Can you work these out from the drawing? Everything is in mm from the part's minimum corner. A direction names the side the tool comes from. Round coordinates to 2 decimals unless told otherwise and drop trailing zeros. Loops run counter-clockwise (first coordinate to the right, second up) from the corner with the lowest first, then second, coordinate; pieces in that order, holes last. Notation, with made-up numbers: M -30,20.5 L -8,20.5 A28 ccw -8,56.5 Z; hole C 66.25,68 d10. An arc over 180 degrees is marked long. Use a Markdown table: item, result.
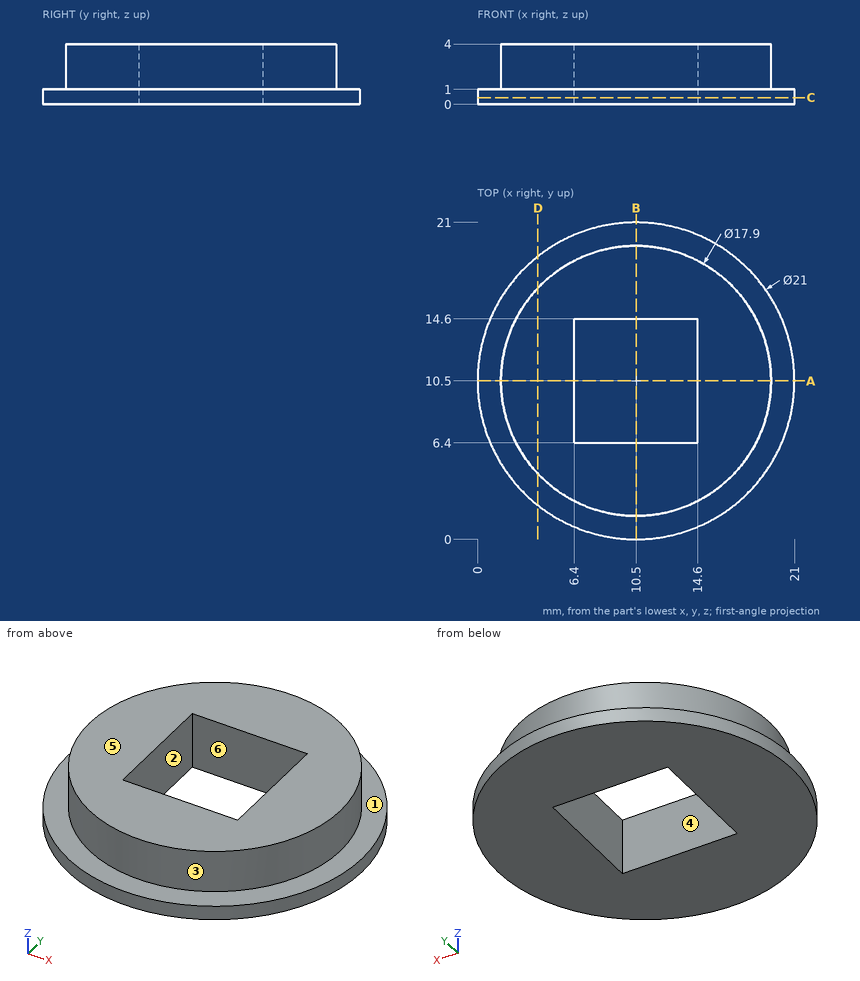
1. We'd pull the mould along X, two halves only. Please class the marked faces 1, 2, 3 and 4: +X half, -X half, draft (parallel to the pull), parting line (faces both ways), or undercut.
Answer sheet:
| item | result |
|---|---|
| face 1 | draft |
| face 2 | undercut |
| face 3 | parting line |
| face 4 | undercut |
2. For pin 1 Ø1.5 at (x, z) = (13, 1) entering from -Y; pin 2 Ø2 at (y, z) = (8.5, 1) entering from -X; pin 3 Ø2 at (x, z) = (18.5, 1.5) entering from +Y, each with a flat end and sliding along its axis, tell me the tip position at first contact or that it passes through.
Answer sheet:
| item | result |
|---|---|
| pin 1 | y = 0.15 |
| pin 2 | x = 0.05 |
| pin 3 | y = 18.2 |
3. Imagine slicing it at C-C, the plane z = 0.45. Write out the boundary of the cut face in (x, y).
Answer sheet:
| item | result |
|---|---|
| outline | C 10.5,10.5 d21; hole M 6.4,6.4 L 14.6,6.4 L 14.6,14.6 L 6.4,14.6 Z |
4. Imagine slicing it at D-D, the plane x = 4. Write out the boundary of the cut face in (y, z), then the cut area to 3 significant figures.
Answer sheet:
| item | result |
|---|---|
| outline | M 2.25,0 L 18.75,0 L 18.75,1 L 16.65,1 L 16.65,4 L 4.35,4 L 4.35,1 L 2.25,1 Z |
| area | 53.4 mm2 |
5. Which directions (+Z, -Z, +X, -X, +Y, -Y) give clear straight access to the entire face, cutting with the end or side of a thin tool? Please do the marked faces 5 and 6.
Answer sheet:
| item | result |
|---|---|
| face 5 | +Z, +X, -X, +Y, -Y |
| face 6 | +Z, -Z |
6. I need wall thicknesses on probe 1 along Y at (x, z) = (14.25, 2.8); probe 2 along Y at (x, z) = (8, 3.1); probe 3 along X at (y, z) = (6.5, 3.2). Which ranges of each line are inside material? Lowest first, please. Write a range as from..to.
Answer sheet:
| item | result |
|---|---|
| probe 1 | 2.37..6.4, 14.6..18.63 |
| probe 2 | 1.91..6.4, 14.6..19.09 |
| probe 3 | 2.49..6.4, 14.6..18.51 |
7. Imagine slicing it at A-A, the plane y = 10.5. Write out the boundary of the cut face in (x, z), then the cut area to 3 significant figures.
Answer sheet:
| item | result |
|---|---|
| outline | M 0,0 L 6.4,0 L 6.4,4 L 1.55,4 L 1.55,1 L 0,1 Z; M 14.6,0 L 21,0 L 21,1 L 19.45,1 L 19.45,4 L 14.6,4 Z |
| area | 41.9 mm2 |
